Check sheet for the modelled part. Datum: model origin and axes. Units: mm. Face numbers are marked on the shaded views. A direction names the side the tool comes from. Round coordinates to 2 decimals unless told otherwise and drop trailing zeros. Write each loop counter-clockwise with the first axis right and the second up, starting at its lowest first coordinate (ties: lowest second). Pieces come first, ordered by that corner, then holes. Notation, with made-up numbers: (-5.5, 1.5) -> (22.5, 1.5) arc R8 ccw to (22.5, 7.5) -> close; hole circle Ø4 at (69.5, -28). An arc over 180 degrees is marked (long way). One line per item, written item: value.
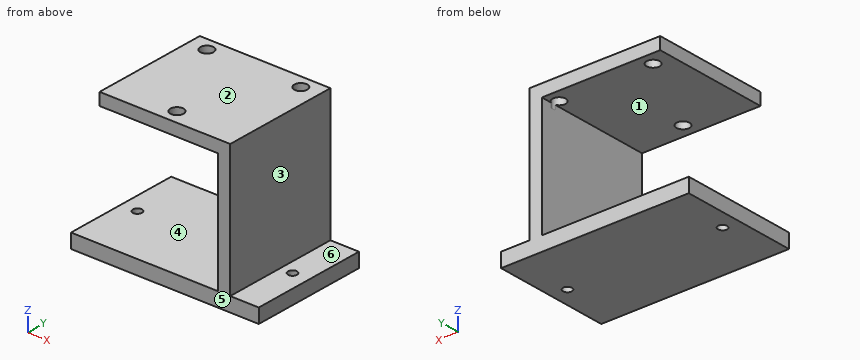
from build123d import *

# Parameters (mm, degrees)
F0_W     = 46
F0_H     = 29
F1_DEPTH = 3.5
F2_W     = 32
F2_H     = 29
F3_DEPTH = 32.25
F4_W     = 29
F4_H     = 29.25
F5_DEPTH = 29
F7_D     = 3.2
F7_DEPTH = 4.1
F7_TIP   = 0.9613769904
F9_D     = 2.2


with BuildPart() as f1:
    # F0 (on Top) → F1 (new body)
    with BuildSketch(Plane.XY):
        Rectangle(F0_W, F0_H)
    extrude(amount=F1_DEPTH)

    # F2 (on face) → F3 (join)
    with BuildSketch(Plane.XY.offset(3.5)):
        Rectangle(F2_W, F2_H)
    extrude(amount=F3_DEPTH)

    # F4 (on face) → F5 (cut)
    with BuildSketch(Plane.XZ.offset(14.5)):
        with Locations((-1.5, 18.125)):
            Rectangle(F4_W, F4_H)
    extrude(amount=-F5_DEPTH, mode=Mode.SUBTRACT)

    # F7
    with Locations(Plane.XY.offset(35.75)):
        with Locations((-11.5, 11.25), (11.5, 11.25), (0, -11)):
            Hole(F7_D / 2, depth=F7_DEPTH)
            with Locations((0, 0, -(F7_DEPTH + F7_TIP / 2))):  # 118° drill point
                Cone(0, F7_D / 2, F7_TIP, mode=Mode.SUBTRACT)

    # F9 (through all)
    with Locations(Plane.XY.offset(3.5)):
        with Locations((-19, 0), (19, 0)):
            Hole(F9_D / 2)


solid = f1.part
Item 1: Sectioned sample at B-B on y = -11. Enter the section's corners in (x, z), and give its area (3 significant figures).
Answer:
outline: (-23, 0) -> (23, 0) -> (23, 3.5) -> (16, 3.5) -> (16, 35.75) -> (1.6, 35.75) -> (1.6, 32.75) -> (13, 32.75) -> (13, 3.5) -> (-23, 3.5) -> close; (-16, 32.75) -> (-1.6, 32.75) -> (-1.6, 35.75) -> (-16, 35.75) -> close
area: 335 mm^2
Item 2: Sectioned sample at C-C on x = 0. Enter the section's corners in (y, z), and give its area (3 significant figures).
Answer:
outline: (-14.5, 0) -> (14.5, 0) -> (14.5, 3.5) -> (-14.5, 3.5) -> close; (-14.5, 32.75) -> (-12.6, 32.75) -> (-12.6, 35.75) -> (-14.5, 35.75) -> close; (-9.4, 32.75) -> (14.5, 32.75) -> (14.5, 35.75) -> (-9.4, 35.75) -> close
area: 179 mm^2
Item 3: Thickness scan on line 1 (Y direction, x = 0, z = 33.55); line 2 (Y direction, x = -19, z = 1.95); line 3 (Z direction, x = -1.5, y = -5.75). Record the ranges inside material, lowest first.
Answer:
line 1: y = -14.5 to -12.6, -9.4 to 14.5
line 2: y = -14.5 to -1.1, 1.1 to 14.5
line 3: z = 0 to 3.5, 32.75 to 35.75
Item 4: Sectioned sample at A-A on y = 11.25. Enter the section's corners in (x, z), and give its area (3 significant figures).
Answer:
outline: (-23, 0) -> (23, 0) -> (23, 3.5) -> (16, 3.5) -> (16, 35.75) -> (13.1, 35.75) -> (13.1, 31.65) -> (13, 31.59) -> (13, 3.5) -> (-23, 3.5) -> close; (-16, 32.75) -> (-13.1, 32.75) -> (-13.1, 35.75) -> (-16, 35.75) -> close; (-9.9, 32.75) -> (9.9, 32.75) -> (9.9, 35.75) -> (-9.9, 35.75) -> close
area: 325 mm^2
Item 5: Sectioned sample at D-D on x = -19. Enter the section's corners in (y, z).
Answer:
outline: (-14.5, 0) -> (-1.1, 0) -> (-1.1, 3.5) -> (-14.5, 3.5) -> close; (1.1, 0) -> (14.5, 0) -> (14.5, 3.5) -> (1.1, 3.5) -> close
Item 6: Depth check by flat-ended pin: P1, Ø5, axis at x = 16, y = 10, coming from the -Z side; P2, Ø2, axis at x = 19, y = -5.5, coming from the +Z side; P3, Ø3.5, axis at y = -2.5, z = 34, coming from the -X side; P4, Ø14.5, axis at y = 6, z = 12.5, coming from the -X side. Enter the tip coordinate at first touch or a pass-through.
Answer:
P1: stops at z = 0
P2: stops at z = 3.5
P3: stops at x = -16
P4: stops at x = 13
Item 7: Mould release check, pull along Z, two halves, no side actions. Record for the marked faces 4, 5 and 6: pulls with the +Z half, pulls with the -Z half, needs draft (parallel to the pull), parting line crosses it, or undercut.
Answer:
face 4: undercut
face 5: needs draft
face 6: pulls with the +Z half
Item 8: Tool access check on the marked faces 1, 2 and 3. Record the directions out of +Z, -Z, +X, -X, +Y, -Y that give a thin tool (end or side, any length) a straight path to the whole face; none if there is none.
Answer:
face 1: -X, +Y, -Y
face 2: +Z, +X, -X, +Y, -Y
face 3: +Z, +X, +Y, -Y
